Read the model definition and answer for the solid it produces. Units are mm, in the model's axes. A direction names the side the tool comes from. Coordinates: 2 decimals unless noted, no trailing zeros. Loops run counter-clockwise (first coordinate to the right, second up) from the corner with the lowest first, then second, coordinate; pieces in that order, holes last. Notation, with made-up numbers: M -26,57.5 L 28,57.5 A26 ccw 28,74.5 Z; hole C -10.75,79.25 d9. An arc over 180 degrees is marked long. Use one line per item in the form item = value. Start each with the question number.
1. A tool of negligible diameter and unlimited length cuts with its end or side. For faces 1 (the flat face through (-55, 0, 0)), 2 (the cylindrical face through (-75.87, -0.31, 3.45)), 3 (the flat face through (-45, 4, 3)), from which of +Z, -Z, +X, -X, +Y, -Y can it reach the whole face along a straight path? Write none if from no direction.
2. The part is cut by section A-A (x = -42.5). Give the vertices of the cut face in (y, z).
3. The part is cut by section D-D (y = 1). Give the number of separate pieces and of enclosed holes in the cut face, plus the area to 3 significant figures.
4. Find the intervals of material crossed by probe 1 along Y at (x, z) = (-68.5, 18.5); probe 2 along Y at (x, z) = (-47.5, 2); probe 3 along X at (y, z) = (1.5, 3), in increasing order. Write a range as [from, to].
5. Flat-ended cylindrical pins translate along their axes: pin 1 (3 mm diameter, centred on x = -46, z = 2, fed in from -Y); pin 2 (5 mm diameter, centred on y = 3.5, z = 11.5, fed in from +X); pin 3 (9 mm diameter, centred on x = -42, y = -1.5, fed in from +Z). Find the tip coordinate at first contact, or state that the pin passes through.
6. The part is cut by section B-B (z = 24). Give the vertices of the cut face in (x, y).
7. For a pull along Y with two mould halves and no side action, classify faces 4 (the flat face through (-42, -2, 3)), 5 (the flat face through (-42, 2, 3)), 6 (the flat face through (-45, -4, 3)), 7 (the flat face through (-65, -4, 32)) as released by +Y, released by -Y, zero draft, split by the parting line, or undercut.
8. The part is cut by section C-C (x = -59). Give the vertices of the cut face in (y, z).
from build123d import *

# Parameters (mm, degrees)
F1_DEPTH    = 6.5
F3_DEPTH    = 25.5
F4_R        = 5
F5_DEPTH    = 32
F6_R        = 7.0774645673
F6_R_2      = 5
F7_DEPTH    = 12
F8_S5_R     = 5
F8_T6_DEPTH = 12


# Not quite as in the source:
# - a fillet or chamfer that OpenCascade refuses, or shapes differently, is made with other operations: its cross-section is extruded or revolved along the edge and cut away or added


with BuildPart() as f1:
    # F0 (on Top) → F1 (new body)
    with BuildSketch(Plane.XY):
        with BuildLine():
            Line((-28.7369439649, 4), (-60.7369439649, 4))
            ThreePointArc((-60.7369439649, 4), (-70.8534266602, 8.7624288794), (-77.7992017132, 0))
            ThreePointArc((-77.7992017132, 0), (-70.8534266602, -8.7624288794), (-60.7369439649, -4))
            Line((-60.7369439649, -4), (-28.7369439649, -4))
            ThreePointArc((-28.7369439649, -4), (-25.9085168402, -2.8284271247), (-24.7369439649, 0))
            ThreePointArc((-24.7369439649, 0), (-25.9085168402, 2.8284271247), (-28.7369439649, 4))
        make_face()
        with BuildLine():
            ThreePointArc((-54.7369439649, 0), (-54.1511575273, 1.4142135624), (-52.7369439649, 2))
            Line((-52.7369439649, 2), (-30.7369439649, 2))
            ThreePointArc((-30.7369439649, 2), (-29.3227304026, 1.4142135624), (-28.7369439649, 0))
            ThreePointArc((-28.7369439649, 0), (-29.3227304026, -1.4142135624), (-30.7369439649, -2))
            Line((-30.7369439649, -2), (-52.7369439649, -2))
            ThreePointArc((-52.7369439649, -2), (-54.1511575273, -1.4142135624), (-54.7369439649, 0))
        make_face(mode=Mode.SUBTRACT)
    extrude(amount=F1_DEPTH)

    # F2 (on face) → F3 (join)
    with BuildSketch(Plane.XY.offset(6.5)):
        with BuildLine():
            ThreePointArc((-60.7369439649, -4), (-60.0367728338, -2.0542249469), (-59.7992017132, 0))
            ThreePointArc((-59.7992017132, 0), (-60.0367728338, 2.0542249469), (-60.7369439649, 4))
            ThreePointArc((-60.7369439649, 4), (-77.7992017132, 0), (-60.7369439649, -4))
        make_face()
    extrude(amount=F3_DEPTH)

    # F4 (on face) → F5 (cut, through all)
    with BuildSketch(Plane.XY.offset(32)):
        with Locations((-68.7992017132, 0)):
            Circle(F4_R)
    extrude(amount=-F5_DEPTH, mode=Mode.SUBTRACT)

    # F6 (on face) → F7 (cut)
    with BuildSketch(Plane(origin=(0, 0, 0), x_dir=(1, 0, 0), z_dir=(0, 0, -1))):
        with Locations((-68.7992017132, 0)):
            Circle(F6_R)
        with Locations((-68.7992017132, 0)):
            Circle(F6_R_2, mode=Mode.SUBTRACT)
    extrude(amount=-F7_DEPTH, mode=Mode.SUBTRACT)

    # F8: chamfer of 5 on 1 edges, made by hand


with BuildPart() as f8_tool2:
    # F8_s3 → F8_t4 (revolve)
    with BuildSketch(Plane.XZ):
        Polygon((-61.721737146, 7), (-66.721737146, 12), (-61.721737146, 12), align=None)
    revolve(axis=Axis((-68.7992017132, 0, 12), (0, 0, -1)))

    # F8_s5 → F8_t6 (cut, symmetric)
    with BuildSketch(Plane.XY.offset(9.5)):
        with Locations((-68.7992017132, 0)):
            Circle(F8_S5_R)
    extrude(amount=F8_T6_DEPTH, both=True, mode=Mode.SUBTRACT)


with BuildPart() as f1_1:
    add(f1.part)

    # F8_t1: union F8_tool2
    add(f8_tool2.part)


solid = f1_1.part
Computed values:
q1.face_1 = -Z, +X, -X, +Y, -Y
q1.face_2 = -Z
q1.face_3 = +Z, -Z, +X, +Y
q2.outline = M -4,0 L -2,0 L -2,6.5 L -4,6.5 Z; M 2,0 L 4,0 L 4,6.5 L 2,6.5 Z
q3.separate_pieces = 3
q3.enclosed_holes = 0
q3.area = 287 mm²
q4.probe_1 = [-9, -4.99], [4.99, 9]
q4.probe_2 = [-4, -2], [2, 4]
q4.probe_3 = [-77.67, -75.72], [-61.88, -54.06], [-29.41, -25.03]
q5.pin_1 = -4
q5.pin_2 = -59.85
q5.pin_3 = 6.5
q6.outline = C -68.8,0 d18; hole C -68.8,0 d10
q7.face_4 = undercut
q7.face_5 = undercut
q7.face_6 = released by -Y
q7.face_7 = zero draft
q8.outline = M -4,0 L 4,0 L 4,6.5 L -4,6.5 Z
